CAD build for the part. Positions are in the model's coordinates, mm. Face numbers are marked on the shaded views. A direction names the side the tool comes from. Round coordinates to 2 decimals unless told otherwise and drop trailing zeros. Order: outer loops, then holes, each group sorted by start corner. A loop starts at its lowest first (then second) coordinate and runs counter-clockwise, first axis right, second up. Notation, with made-up numbers: (65, 86.25) -> (98, 86.25) arc R31 cw to (98, 120.25) -> close; hole circle Ø5 at (47.5, 53.25). An arc over 180 degrees is marked (long way). Return JSON: item names as keys, results as strings. Group by question number.
Q1. Probe line 1 along X through (y, z) = (-300.5, 9.5); line 2 along Z through (x, y) = (845, -104); line 3 along X through (y, z) = (-119.5, 2.5). List the from-to ranges inside material, lowest first.
Q2. Cut at C-C (z = 11.5). Write the cut outline in (x, y).
Q3. Cut at B-B (x = 919.5). Write the cut outline in (y, z).
Q4. Flat gauge pins, fed straight in: pin 1 (12 mm diameter, centred on x = 988, y = -152.5, fed in from +Z); pin 2 (2 mm diameter, centred on y = -188, z = 4.5, fed in from +X); pin 3 (1.6 mm diameter, centred on y = -149.5, z = 1, fed in from -X). Where does each tip first touch, or does it go through?
Q5. Which spindle directions (+Z, -Z, +X, -X, +Y, -Y) get a long thin tool onto all of the face, cutting with end or side? Do the marked faces 1 and 2. Say none if no direction does.
Q6. Cut at D-D (x = 791). Write the cut outline in (y, z).
Q7. Cut at A-A (y = -266.5). Count the separate pieces of the cut face and the enclosed holes in it, then the cut area to 3 significant figures.
from build123d import *

# Parameters (mm, degrees)
SKETCH_1_W            = 280
SKETCH_1_H            = 350
EXTRUDE_1_DEPTH       = 2
SKETCH_2_W            = 1.551264613
SKETCH_2_H            = 30
EXTRUDE_2_DEPTH       = 350
EXTRUDE_3_DEPTH       = 350
SKETCH_3_R            = 2.5
CUT_EXTRUDE_1_DEPTH   = 1119.062393976
SHEET_START           = -330.973817188
SHEET_METAL_1_DEPTH   = 350
SHEET_METAL_1_2_DEPTH = 350
SKETCH_29_R           = 2.25
CUT_EXTRUDE_3_DEPTH   = 10
FILLET_1_R            = 10


# Read off the part's stored shape, not the designer's step: 솔리드-변환1
with BuildPart() as part:
    # 스케치1 → 보스-돌출1 (new body)
    with BuildSketch(Plane.XY):
        with Locations((905.507072504, -155.973817188)):
            Rectangle(SKETCH_1_W, SKETCH_1_H)
    extrude(amount=EXTRUDE_1_DEPTH)

    # 스케치2 → 보스-돌출2 (add)
    with BuildSketch(Plane(origin=(0, 19.026182812, 0), x_dir=(1, 0, 0), z_dir=(0, 1, 0))):
        with Locations((766.282704811, -17)):
            Rectangle(SKETCH_2_W, SKETCH_2_H)
    extrude(amount=-EXTRUDE_2_DEPTH)

    # 스케치10 → 보스-돌출3 (add)
    with BuildSketch(Plane(origin=(0, 19.026182812, 0), x_dir=(1, 0, 0), z_dir=(0, 1, 0))):
        Polygon((767.058337117, -2), (768.508337117, -2), (768.508337117, -6.001264612), (768.508337117, -32), (767.058337117, -32), align=None)
    extrude(amount=-EXTRUDE_3_DEPTH)

    # 스케치3 → 컷-돌출1 (cut, through all)
    with BuildSketch(Plane(origin=(1.179072504, 0, -191.38056669), x_dir=(1, 0, 0), z_dir=(0, 0, -1))):
        with Locations(Location((1034.328, 255.973817188, 0), (0, 0, 180))):
            Circle(SKETCH_3_R)
        with Locations(Location((1034.328, 55.973817188, 0), (0, 0, 180))):
            Circle(SKETCH_3_R)
        with Locations(Location((864.328, -9.026182812, 0), (0, 0, 180))):
            Circle(SKETCH_3_R)
        with Locations(Location((814.328, -9.026182812, 0), (0, 0, 180))):
            Circle(SKETCH_3_R)
        with Locations(Location((864.328, 320.973817188, 0), (0, 0, 180))):
            Circle(SKETCH_3_R)
        with Locations(Location((814.328, 320.973817188, 0), (0, 0, 180))):
            Circle(SKETCH_3_R)
        with Locations(Location((1034.328, 290.973817188, 0), (0, 0, 180))):
            Circle(SKETCH_3_R)
        with Locations(Location((1034.328, 20.973817188, 0), (0, 0, 180))):
            Circle(SKETCH_3_R)
        with Locations(Location((934.328, 320.973817188, 0), (0, 0, 180))):
            Circle(SKETCH_3_R)
        with Locations(Location((934.328, -9.026182812, 0), (0, 0, 180))):
            Circle(SKETCH_3_R)
        with Locations(Location((1034.328, 88.973817188, 0), (0, 0, 180))):
            Circle(SKETCH_3_R)
        with Locations(Location((1034.328, 222.973817188, 0), (0, 0, 180))):
            Circle(SKETCH_3_R)
    extrude(amount=-CUT_EXTRUDE_1_DEPTH, mode=Mode.SUBTRACT)

    # Sheet Metal 1 outline → Sheet Metal 1 (cut)
    with BuildSketch(Plane(origin=(0, 0, 0), x_dir=(1, 0, 0), z_dir=(0, 1, 0)).offset(SHEET_START)):
        with BuildLine():
            Line((765.507072504, -32), (766.508337117, -32))
            Line((766.508337117, -32), (766.508337117, -4))
            ThreePointArc((766.508337117, -4), (767.679909992, -1.171572875), (770.508337117, 0))
            Line((770.508337117, 0), (765.507072504, 0))
            Line((765.507072504, 0), (765.507072504, -32))
        make_face()
    extrude(amount=SHEET_METAL_1_DEPTH, mode=Mode.SUBTRACT)

    # Sheet Metal 1 2 outline → Sheet Metal 1 2 (add)
    with BuildSketch(Plane(origin=(0, 0, 0), x_dir=(1, 0, 0), z_dir=(0, 1, 0)).offset(SHEET_START)):
        with BuildLine():
            ThreePointArc((768.508337117, -4), (769.094123555, -2.585786438), (770.508337117, -2))
            Line((770.508337117, -2), (768.508337117, -2))
            Line((768.508337117, -2), (768.508337117, -4))
        make_face()
    extrude(amount=SHEET_METAL_1_2_DEPTH)

    # 스케치29 → 컷-돌출3 (cut)
    with BuildSketch(Plane.XY.offset(2)):
        with Locations((945.507072504, -103.473817188)):
            Circle(SKETCH_29_R)
        with Locations((945.507072504, -208.473817188)):
            Circle(SKETCH_29_R)
        with Locations((840.507072504, -103.473817188)):
            Circle(SKETCH_29_R)
        with Locations((840.507072504, -208.473817188)):
            Circle(SKETCH_29_R)
        with BuildLine():
            Line((1015.507072504, -40.973817188), (1015.507072504, -270.973817188))
            ThreePointArc((1015.507072504, -270.973817188), (1002.507072504, -283.973817188), (989.507072504, -270.973817188))
            Line((989.507072504, -270.973817188), (989.507072504, -40.973817188))
            ThreePointArc((989.507072504, -40.973817188), (1002.507072504, -27.973817188), (1015.507072504, -40.973817188))
        make_face()
        with BuildLine():
            Line((977.507072504, -40.973817188), (977.507072504, -270.973817188))
            ThreePointArc((977.507072504, -270.973817188), (964.507072504, -283.973817188), (951.507072504, -270.973817188))
            Line((951.507072504, -270.973817188), (951.507072504, -40.973817188))
            ThreePointArc((951.507072504, -40.973817188), (964.507072504, -27.973817188), (977.507072504, -40.973817188))
        make_face()
        with BuildLine():
            Line((939.507072504, -40.973817188), (939.507072504, -270.973817188))
            ThreePointArc((939.507072504, -270.973817188), (926.507072504, -283.973817188), (913.507072504, -270.973817188))
            Line((913.507072504, -270.973817188), (913.507072504, -40.973817188))
            ThreePointArc((913.507072504, -40.973817188), (926.507072504, -27.973817188), (939.507072504, -40.973817188))
        make_face()
        with BuildLine():
            Line((906.507072504, -40.973817188), (906.507072504, -270.973817188))
            ThreePointArc((906.507072504, -270.973817188), (893.507072504, -283.973817188), (880.507072504, -270.973817188))
            Line((880.507072504, -270.973817188), (880.507072504, -40.973817188))
            ThreePointArc((880.507072504, -40.973817188), (893.507072504, -27.973817188), (906.507072504, -40.973817188))
        make_face()
        with BuildLine():
            Line((873.507072504, -40.973817188), (873.507072504, -270.973817188))
            ThreePointArc((873.507072504, -270.973817188), (860.507072504, -283.973817188), (847.507072504, -270.973817188))
            Line((847.507072504, -270.973817188), (847.507072504, -40.973817188))
            ThreePointArc((847.507072504, -40.973817188), (860.507072504, -27.973817188), (873.507072504, -40.973817188))
        make_face()
        with BuildLine():
            Line((833.507072504, -40.973817188), (833.507072504, -270.973817188))
            ThreePointArc((833.507072504, -270.973817188), (820.507072504, -283.973817188), (807.507072504, -270.973817188))
            Line((807.507072504, -270.973817188), (807.507072504, -40.973817188))
            ThreePointArc((807.507072504, -40.973817188), (820.507072504, -27.973817188), (833.507072504, -40.973817188))
        make_face()
    extrude(amount=-CUT_EXTRUDE_3_DEPTH, mode=Mode.SUBTRACT)

    # 필렛1
    fillet_1_edges = [part.edges().sort_by_distance(p)[0] for p in [
        (1045.507072504, 19.026182812, 1),
        (1045.507072504, -330.973817188, 1),
        (767.508337117, -330.973817188, 32),
        (767.508337117, 19.026182812, 32),
    ]]
    fillet(fillet_1_edges, radius=FILLET_1_R)


solid = part.part
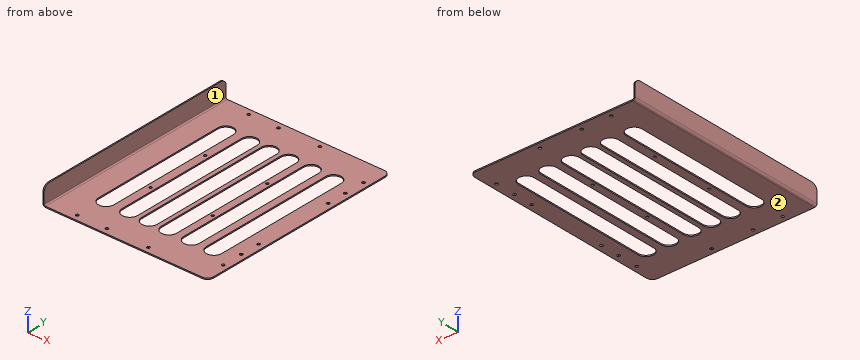
Solution:
{
 "1": {"line 1": "x = 766.51 to 768.51", "line 2": "z = 0 to 2", "line 3": "x = 766.8 to 769.19"},
 "2": {"outline": "(766.51, -330.97) -> (768.51, -330.97) -> (768.51, 19.03) -> (766.51, 19.03) -> close"},
 "3": {"outline": "(-330.97, 0) -> (-281.92, 0) -> (-281.92, 2) -> (-330.97, 2) -> close; (-30.02, 0) -> (19.03, 0) -> (19.03, 2) -> (-30.02, 2) -> close"},
 "4": {"pin 1": "stops at z = 2", "pin 2": "stops at x = 768.57", "pin 3": "stops at x = 767.17"},
 "5": {"face 1": "+Z, +X, +Y, -Y", "face 2": "-Z, +X, -X, +Y, -Y"},
 "6": {"outline": "(-330.97, 0) -> (19.03, 0) -> (19.03, 2) -> (-330.97, 2) -> close"},
 "7": {"separate pieces": "7", "enclosed holes": "0", "area": "303 mm²"}
}
